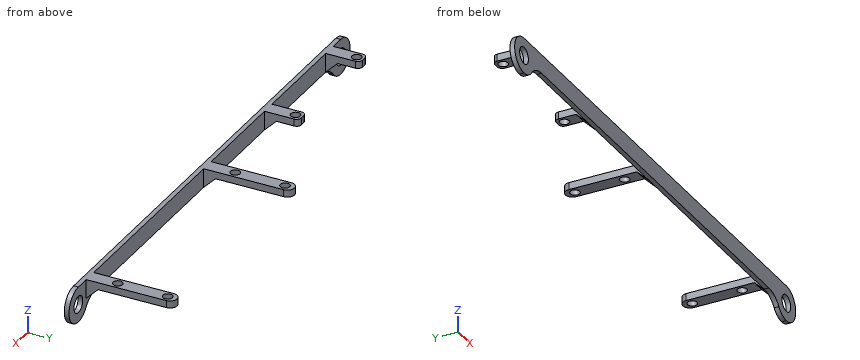
```python
from build123d import *

# Parameters (mm, degrees)
SKETCH1_R           = 3.5
BOSS_EXTRUDE1_DEPTH = 2
SKETCH2_W           = 6
SKETCH2_H           = 36.75
SKETCH2_R           = 2
SKETCH2_H_2         = 14.5
BOSS_EXTRUDE2_DEPTH = 3
FILLET1_RADIUS      = 3
FILLET1_LENGTH      = 3
FILLET2_RADIUS      = 3
FILLET2_LENGTH      = 3
FILLET3_R           = 2
CHAMFER1_SIZE       = 5
CUT_EXTRUDE1_START  = -10
CUT_EXTRUDE1_DEPTH  = 10
FILLET4_R           = 10


with BuildPart() as part:
    # Sketch1 → Boss-Extrude1 (new body)
    with BuildSketch(Plane(origin=(0, -82.5, 0), x_dir=(1, 0, 0), z_dir=(0, 1, 0))):
        with BuildLine():
            Line((-105, 67.5), (105, 67.5))
            ThreePointArc((105, 67.5), (112.5, 60), (105, 52.5))
            Line((105, 52.5), (-105, 52.5))
            ThreePointArc((-105, 52.5), (-112.5, 60), (-105, 67.5))
        make_face()
        with Locations(Location((-105, 60, 0), (0, 0, 270))):
            Circle(SKETCH1_R, mode=Mode.SUBTRACT)
        with Locations(Location((105, 60, 0), (0, 0, 270))):
            Circle(SKETCH1_R, mode=Mode.SUBTRACT)
    extrude(amount=BOSS_EXTRUDE1_DEPTH)

    # Sketch2 → Boss-Extrude2 (add)
    # profile 1 of 4: a face of its own
    with BuildSketch(Plane(origin=(0, 0, -52.5), x_dir=(-1, 0, 0), z_dir=(0, 0, -1))):
        with Locations((-95.704993888, -62.125)):
            Rectangle(SKETCH2_W, SKETCH2_H)
        with Locations((-95.704993888, -47.75)):
            Circle(SKETCH2_R, mode=Mode.SUBTRACT)
        with Locations((-95.704993888, -68.75)):
            Circle(SKETCH2_R, mode=Mode.SUBTRACT)
    # profile 2 of 4: a face of its own
    with BuildSketch(Plane(origin=(0, 0, -52.5), x_dir=(-1, 0, 0), z_dir=(0, 0, -1))):
        with Locations((-1.704993888, -62.125)):
            Rectangle(SKETCH2_W, SKETCH2_H)
        with Locations((-1.704993888, -47.75)):
            Circle(SKETCH2_R, mode=Mode.SUBTRACT)
        with Locations((-1.704993888, -68.75)):
            Circle(SKETCH2_R, mode=Mode.SUBTRACT)
    # profile 3 of 4: a face of its own
    with BuildSketch(Plane(origin=(0, 0, -52.5), x_dir=(-1, 0, 0), z_dir=(0, 0, -1))):
        with Locations((47.003472144, -73.25)):
            Rectangle(SKETCH2_W, SKETCH2_H_2)
        with Locations((47.003472144, -69)):
            Circle(SKETCH2_R, mode=Mode.SUBTRACT)
    # profile 4 of 4: a face of its own
    with BuildSketch(Plane(origin=(0, 0, -52.5), x_dir=(-1, 0, 0), z_dir=(0, 0, -1))):
        with Locations((96.003472144, -73.25)):
            Rectangle(SKETCH2_W, SKETCH2_H_2)
        with Locations((96.003472144, -69)):
            Circle(SKETCH2_R, mode=Mode.SUBTRACT)
    extrude(amount=BOSS_EXTRUDE2_DEPTH)

    # Fillet1: full round fillet: the end face becomes a half cylinder, R = half its width
    fillet1_face = Plane((95.704993888, -43.75, -54), x_dir=(0, 0, -1), z_dir=(0, 1, 0))  # on the end face: x along it, z out of the body
    fillet1_slab = fillet1_face.offset(-FILLET1_RADIUS / 2) * Box(FILLET1_LENGTH, 2 * FILLET1_RADIUS, FILLET1_RADIUS, mode=Mode.PRIVATE)  # the body's end, R deep
    fillet1_round = Plane((95.704993888, -46.75, -54), x_dir=(0, 1, 0), z_dir=(0, 0, -1)) * Cylinder(FILLET1_RADIUS, FILLET1_LENGTH, mode=Mode.PRIVATE)  # its axis R under the face
    add(fillet1_slab - fillet1_round, mode=Mode.SUBTRACT)

    # Fillet2: full round fillet: the end face becomes a half cylinder, R = half its width
    fillet2_face = Plane((1.704993888, -43.75, -54), x_dir=(0, 0, -1), z_dir=(0, 1, 0))  # on the end face: x along it, z out of the body
    fillet2_slab = fillet2_face.offset(-FILLET2_RADIUS / 2) * Box(FILLET2_LENGTH, 2 * FILLET2_RADIUS, FILLET2_RADIUS, mode=Mode.PRIVATE)  # the body's end, R deep
    fillet2_round = Plane((1.704993888, -46.75, -54), x_dir=(0, 1, 0), z_dir=(0, 0, -1)) * Cylinder(FILLET2_RADIUS, FILLET2_LENGTH, mode=Mode.PRIVATE)  # its axis R under the face
    add(fillet2_slab - fillet2_round, mode=Mode.SUBTRACT)

    # Fillet3
    fillet3_edges = [part.edges().sort_by_distance(p)[0] for p in [
        (-44.003472144, -66, -54),
        (-50.003472144, -66, -54),
        (-99.003472144, -66, -54),
        (-93.003472144, -66, -54),
    ]]
    fillet(fillet3_edges, radius=FILLET3_R)

    # Chamfer1
    chamfer1_edges = [part.edges().sort_by_distance(p)[0] for p in [
        (95.704993888, -80.5, -55.5),
        (1.704993888, -80.5, -55.5),
        (-47.003472144, -80.5, -55.5),
        (-96.003472144, -80.5, -55.5),
    ]]
    chamfer(chamfer1_edges, length=CHAMFER1_SIZE)

    # Sketch3 → Cut-Extrude1 (cut)
    with BuildSketch(Plane(origin=(0, -80.5, 0), x_dir=(1, 0, 0), z_dir=(0, 1, 0)).offset(CUT_EXTRUDE1_START)):
        with BuildLine():
            Line((92.704993888, 60.5), (97.516685226, 60.5))
            ThreePointArc((97.516685226, 60.5), (99.876524617, 65.477225575), (105, 67.5))
            Line((105, 67.5), (-105, 67.5))
            ThreePointArc((-105, 67.5), (-99.876524617, 65.477225575), (-97.516685226, 60.5))
            Line((-97.516685226, 60.5), (-93.003472144, 60.5))
            Line((-93.003472144, 60.5), (-50.003472144, 60.5))
            Line((-50.003472144, 60.5), (-44.003472144, 60.5))
            Line((-44.003472144, 60.5), (-1.295006112, 60.5))
            Line((-1.295006112, 60.5), (4.704993888, 60.5))
            Line((4.704993888, 60.5), (92.704993888, 60.5))
        make_face()
    extrude(amount=CUT_EXTRUDE1_DEPTH, mode=Mode.SUBTRACT)

    # Fillet4
    # the kernel refuses this fillet: 10 mm, written as the material it adds along each edge
    with BuildSketch(Plane(origin=(97.516685226, -82.5, -60.5), x_dir=(-1, 0, 0), z_dir=(0, 1, 0))) as fillet4_piece_1_section:
        with BuildLine():
            CenterArc((6.516685226, -10), FILLET4_R, 90, 53.130102354)
            ThreePointArc((-1.483314774, -4), (-0.451249336, -2.107691638), (0, 0))
            Line((0, 0), (6.516685226, 0))
        make_face()
    fillet4_piece_1 = extrude(amount=2, mode=Mode.PRIVATE)
    fillet4_piece_1 = split(fillet4_piece_1, bisect_by=Plane(origin=(95.39414114, -81.261061564, -61.261061564), z_dir=(0, -0.7071067811865476, 0.7071067811865476)), keep=Keep.TOP, mode=Mode.PRIVATE)
    add(fillet4_piece_1)
    with BuildSketch(Plane(origin=(97.516685226, -82.5, -60.5), x_dir=(-1, 0, 0), z_dir=(0, 1, 0))) as fillet4_piece_2_section:
        with BuildLine():
            CenterArc((6.516685226, -10), FILLET4_R, 90, 53.130102354)
            ThreePointArc((-1.483314774, -4), (-0.451249336, -2.107691638), (0, 0))
            Line((0, 0), (6.516685226, 0))
        make_face()
    fillet4_piece_2 = extrude(amount=2, mode=Mode.PRIVATE)
    fillet4_piece_2 = split(fillet4_piece_2, bisect_by=Plane(origin=(97.181808866, -81.694028368, -61.694028368), z_dir=(0, 0.7071067811865476, -0.7071067811865476)), keep=Keep.TOP, mode=Mode.PRIVATE)
    add(fillet4_piece_2)
    with BuildSketch(Plane(origin=(-97.516685226, -82.5, -60.5), x_dir=(1, 0, 0), z_dir=(0, 1, 0))) as fillet4_piece_3_section:
        with BuildLine():
            CenterArc((6.516685226, 10), FILLET4_R, 216.869897646, 53.130102354)
            ThreePointArc((-1.483314774, 4), (-0.451249336, 2.107691638), (0, 0))
            Line((0, 0), (6.516685226, 0))
        make_face()
    fillet4_piece_3 = extrude(amount=2, mode=Mode.PRIVATE)
    fillet4_piece_3 = split(fillet4_piece_3, bisect_by=Plane(origin=(-95.39414114, -81.261061564, -61.261061564), z_dir=(0, -0.7071067811865476, 0.7071067811865476)), keep=Keep.TOP, mode=Mode.PRIVATE)
    add(fillet4_piece_3)
    with BuildSketch(Plane(origin=(-97.516685226, -82.5, -60.5), x_dir=(1, 0, 0), z_dir=(0, 1, 0))) as fillet4_piece_4_section:
        with BuildLine():
            CenterArc((6.516685226, 10), FILLET4_R, 216.869897646, 53.130102354)
            ThreePointArc((-1.483314774, 4), (-0.451249336, 2.107691638), (0, 0))
            Line((0, 0), (6.516685226, 0))
        make_face()
    fillet4_piece_4 = extrude(amount=2, mode=Mode.PRIVATE)
    fillet4_piece_4 = split(fillet4_piece_4, bisect_by=Plane(origin=(-97.181808866, -81.694028368, -61.694028368), z_dir=(0, 0.7071067811865476, -0.7071067811865476)), keep=Keep.TOP, mode=Mode.PRIVATE)
    add(fillet4_piece_4)


solid = part.part
```
Model file for the job. Use its own axes, mm. Coordinates: 2 decimals unless noted, no trailing zeros. Write each loop counter-clockwise with the first axis right and the second up, starting at its lowest first coordinate (ties: lowest second). Pieces come first, ordered by that corner, then holes. Notation, with made-up numbers: (13, 19) - (64, 19) arc R18 cw to (64, 43) - close; hole circle Ø6 at (25.25, 7). An arc over 180 degrees is marked (long way). Use a Markdown table: item, result. Add a question column.
Item 1: Band-saw the part on A-A, the plane y = -64. Write the cut outline in (x, z) (3 decimals), and give its area (3 significant figures).
Item 2: Band-saw the part on B-B, the plane x = -61. Write the cut outline in (y, z), and give its area (3 significant figures).
Item 3: Drop flat-ended pins along their axis: pin 1 (4 mm diameter, centred on x = -17.5, z = -56.5, fed in from +Y); pin 2 (2.5 mm diameter, centred on x = 1.7, y = -68.75, fed in from -Z) (3 decimals); pin 3 (9 mm diameter, centred on y = -77, z = -55.5, fed in from -X); pin 4 (3 mm diameter, centred on x = 0, z = -58, fed in from +Y). Give the stop position or say it passes through.
Item 4: Drill centre lines: line 1 along X through (y, z) = (-81.95, -60); line 2 along X through (y, z) = (-62.5, -55.25) (3 decimals); line 3 along Y through (x, z) = (22, -56.5). Where is each one in solid material? Low to high.
A:
| question | item | result |
|---|---|---|
| 1 | outline | (-1.295, -55.5) - (4.705, -55.5) - (4.705, -52.5) - (-1.295, -52.5) - close; (92.705, -55.5) - (98.705, -55.5) - (98.705, -52.5) - (92.705, -52.5) - close |
| 1 | area | 36.0 mm² |
| 2 | outline | (-82.5, -60.5) - (-80.5, -60.5) - (-80.5, -52.5) - (-82.5, -52.5) - close |
| 2 | area | 16.0 mm² |
| 3 | pin 1 | stops at y = -80.5 |
| 3 | pin 2 | passes through |
| 3 | pin 3 | stops at x = -112.31 |
| 3 | pin 4 | stops at y = -76.5 |
| 4 | line 1 | x = -112.5 to -108.5, -101.5 to 101.5, 108.5 to 112.5 |
| 4 | line 2 | x = -1.295 to 4.705, 92.705 to 98.705 |
| 4 | line 3 | y = -82.5 to -80.5 |
